Design review of the part built by this model. Coordinates are the model's own, in mm. Face numbers are marked on the shaded views. Coordinates: 2 decimals unless noted, no trailing zeros. Loops run counter-clockwise (first coordinate to the right, second up) from the corner with the lowest first, then second, coordinate; pieces in that order, holes last. Notation, with made-up numbers: (19.5, 18.5) - (51.5, 18.5) arc R15 cw to (51.5, 37.5) - close; hole circle Ø10 at (75.25, -25). An arc over 180 degrees is marked (long way). Answer in a Markdown table with one row per item. Add a question column.
(1) The part is to be moulded in two halves that separate along Z. For the marked faces 1 and 2, say which applies: released by +Z, released by -Z, zero draft, split by the parting line, or undercut.
(2) We need section C-C, the plane x = 0. Write out the cut boundary in (y, z), plus the area to 3 significant figures.
(3) To check wall thickness, follow L1, parallel to X at y = 2.35, z = -34.5; L2, parallel to X at y = 6.5, z = 44; L3, parallel to Z at x = 35, y = 1.35. State the ranges of each line that lie inside material, in increasing order. Write a range as [from, to].
(4) Clearance check with flat-ended pins moving along their axes: pin 1 (4 mm diameter, centred on x = 56, z = -13, fed in from -Y); pin 2 (12 mm diameter, centred on x = 34, z = -31, fed in from +Y). State where each tip first meets the part, or that it passes through.
(5) We need section A-A, the plane z = -34.5. Write out the cut boundary in (x, y), plus the area to 3 significant figures.
(6) We need section D-D, the plane z = 39.5. Write out the cut boundary in (x, y), plus the area to 3 significant figures.
(7) We need section B-B, the plane y = 4.5. Write out the cut boundary in (x, z).
from build123d import *

# Parameters (mm, degrees)
BOSS_EXTRU_1_DEPTH      = 10
ENL_V_MAT_EXTRU_1_DEPTH = 7
D_GAGEMENT_M41_D        = 4.5
D_GAGEMENT_M41_DEPTH    = 10
D_GAGEMENT_M41_TIP      = 1.351936393


with BuildPart() as part:
    # Esquisse2 → Boss.-Extru.1 (new body)
    with BuildSketch(Plane(origin=(0, 0, 0), x_dir=(1, 0, 0), z_dir=(0, 1, 0))):
        with BuildLine():
            Line((-80, 102.5), (80, 102.5))
            ThreePointArc((80, 102.5), (87.071067812, 99.571067812), (90, 92.5))
            Line((90, 92.5), (90, -92.5))
            ThreePointArc((90, -92.5), (87.071067812, -99.571067812), (80, -102.5))
            Line((80, -102.5), (-80, -102.5))
            ThreePointArc((-80, -102.5), (-87.071067812, -99.571067812), (-90, -92.5))
            Line((-90, -92.5), (-90, 92.5))
            ThreePointArc((-90, 92.5), (-87.071067812, 99.571067812), (-80, 102.5))
        make_face()
    extrude(amount=BOSS_EXTRU_1_DEPTH)

    # Esquisse3 → Enlèv. mat.-Extru.1 (cut)
    with BuildSketch(Plane(origin=(0, 10, 0), x_dir=(1, 0, 0), z_dir=(0, 1, 0))):
        with BuildLine():
            Line((-35, -8.185360488), (-35, -58.185360488))
            ThreePointArc((-35, -58.185360488), (-32.071067812, -65.2564283), (-25, -68.185360488))
            Line((-25, -68.185360488), (25, -68.185360488))
            ThreePointArc((25, -68.185360488), (32.071067812, -65.2564283), (35, -58.185360488))
            Line((35, -58.185360488), (35, -8.185360488))
            ThreePointArc((35, -8.185360488), (0, 89.7), (-35, -8.185360488))
        make_face()
    extrude(amount=-ENL_V_MAT_EXTRU_1_DEPTH, mode=Mode.SUBTRACT)

    # Dégagement M41
    with Locations(Plane(origin=(0, 0, 0), x_dir=(-1, 0, 0), z_dir=(0, -1, 0))):
        with Locations((35, 34.5), (-35, 34.5)):
            Hole(D_GAGEMENT_M41_D / 2, depth=D_GAGEMENT_M41_DEPTH)
            with Locations((0, 0, -(D_GAGEMENT_M41_DEPTH + D_GAGEMENT_M41_TIP / 2))):  # 118° drill point
                Cone(0, D_GAGEMENT_M41_D / 2, D_GAGEMENT_M41_TIP, mode=Mode.SUBTRACT)


solid = part.part
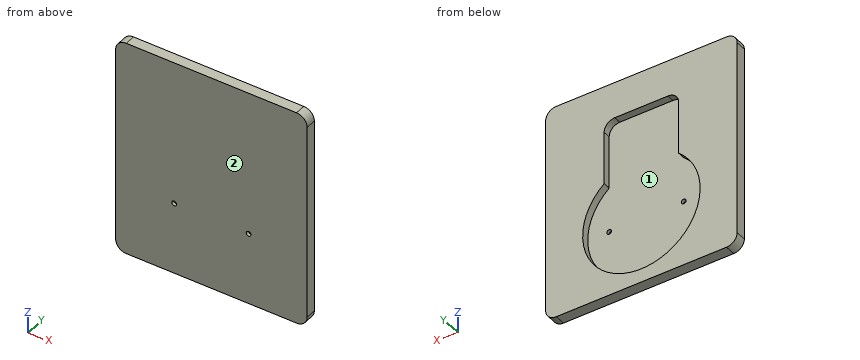
Responses:
| question | item | result |
|---|---|---|
| 1 | face 1 | undercut |
| 1 | face 2 | zero draft |
| 2 | outline | (0, -102.5) - (10, -102.5) - (10, -89.7) - (3, -89.7) - (3, 68.19) - (10, 68.19) - (10, 102.5) - (0, 102.5) - close |
| 2 | area | 945 mm2 |
| 3 | L1 | x = [-90, -37.25], [-32.75, 32.75], [37.25, 90] |
| 3 | L2 | x = [-90, -35], [35, 90] |
| 3 | L3 | z = [-102.5, -36.75], [-32.25, 102.5] |
| 4 | pin 1 | stops at y = 0 |
| 4 | pin 2 | stops at y = 3 |
| 5 | outline | (-90, 0) - (-37.25, 0) - (-37.25, 3) - (-55.2, 3) - (-55.2, 10) - (-90, 10) - close; (-32.75, 0) - (32.75, 0) - (32.75, 3) - (-32.75, 3) - close; (37.25, 0) - (90, 0) - (90, 10) - (55.2, 10) - (55.2, 3) - (37.25, 3) - close |
| 5 | area | 1,000 mm2 |
| 6 | outline | (-90, 0) - (90, 0) - (90, 10) - (35, 10) - (35, 3) - (-35, 3) - (-35, 10) - (-90, 10) - close |
| 6 | area | 1,310 mm2 |
| 7 | outline | (-90, -92.5) arc R10 ccw to (-80, -102.5) - (80, -102.5) arc R10 ccw to (90, -92.5) - (90, 92.5) arc R10 ccw to (80, 102.5) - (-80, 102.5) arc R10 ccw to (-90, 92.5) - close; hole (-35, 8.19) arc R55.2 ccw (long way) to (35, 8.19) - (35, 58.19) arc R10 ccw to (25, 68.19) - (-25, 68.19) arc R10 ccw to (-35, 58.19) - close |
